from build123d import *

# Parameters (mm, degrees)
Y_KSEKLIK_EKSTR_ZYON1_DEPTH      = 0.1
Y_KSEKLIK_EKSTR_ZYON1_DEPTH_BACK = 16.34
IZIM1_R                          = 1.3
IZIM2_R                          = 2
Y_KSEKLIK_EKSTR_ZYON2_DEPTH      = 0.4
Y_KSEKLIK_EKSTR_ZYON3_START      = 0.4
IZIM3_R                          = 2
Y_KSEKLIK_EKSTR_ZYON3_DEPTH      = 0.4
IZIM4_R                          = 0.45
KES_EKSTR_ZYON1_DEPTH            = 0.5
PAH1_SIZE                        = 0.4
KES_EKSTR_ZYON2_START            = -0.5
IZIM5_R                          = 0.45
KES_EKSTR_ZYON2_DEPTH            = 0.5
PAH2_SIZE                        = 0.4


with BuildPart() as part:
    # Çizim1 → Yükseklik-Ekstrüzyon1 (new, two sides: drawn at the far end of the back side and taken through both)
    with BuildSketch(Plane.XY.offset(-Y_KSEKLIK_EKSTR_ZYON1_DEPTH_BACK)):
        with Locations((3.3, -31.281939442)):
            Circle(IZIM1_R)
    extrude(amount=Y_KSEKLIK_EKSTR_ZYON1_DEPTH + Y_KSEKLIK_EKSTR_ZYON1_DEPTH_BACK)

    # Çizim2 → Yükseklik-Ekstrüzyon2 (add)
    with BuildSketch(Plane.XY.offset(0.1)):
        with Locations((3.3, -31.281939442)):
            Circle(IZIM2_R)
    extrude(amount=Y_KSEKLIK_EKSTR_ZYON2_DEPTH)

    # Çizim3 → Yükseklik-Ekstrüzyon3 (add)
    with BuildSketch(Plane(origin=(0, 0, -16.34), x_dir=(-1, 0, 0), z_dir=(0, 0, -1)).offset(Y_KSEKLIK_EKSTR_ZYON3_START)):
        with Locations(Location((-3.3, -31.281939442, 0), (0, 0, 180))):
            Circle(IZIM3_R)
    extrude(amount=-Y_KSEKLIK_EKSTR_ZYON3_DEPTH)

    # Çizim4 → Kes-Ekstrüzyon1 (cut)
    with BuildSketch(Plane(origin=(0, 0, -16.74), x_dir=(-1, 0, 0), z_dir=(0, 0, -1))):
        with Locations((-3.3, -31.281939442)):
            Circle(IZIM4_R)
    extrude(amount=-KES_EKSTR_ZYON1_DEPTH, mode=Mode.SUBTRACT)

    # Pah1
    pah1_edges = [part.edges().sort_by_distance(p)[0] for p in [
        (3.75, -31.281939442, -16.24),
    ]]
    chamfer(pah1_edges, length=PAH1_SIZE)

    # Çizim5 → Kes-Ekstrüzyon2 (cut)
    with BuildSketch(Plane.XY.offset(0.5).offset(KES_EKSTR_ZYON2_START)):
        with Locations(Location((3.3, -31.281939442, 0), (0, 0, 180))):
            Circle(IZIM5_R)
    extrude(amount=KES_EKSTR_ZYON2_DEPTH, mode=Mode.SUBTRACT)

    # Pah2
    pah2_edges = [part.edges().sort_by_distance(p)[0] for p in [
        (3.75, -31.281939442, 0),
    ]]
    chamfer(pah2_edges, length=PAH2_SIZE)


solid = part.part
Verification items for the finished model (mm, model axes). A direction names the side the tool comes from. Coordinates: 2 decimals unless noted, no trailing zeros. Write each loop counter-clockwise with the first axis right and the second up, starting at its lowest first coordinate (ties: lowest second). Pieces come first, ordered by that corner, then holes. Notation, with made-up numbers: M -5.5,9.25 L 17.5,9.25 A18 cw 17.5,22.25 Z; hole C -36,-7 d3. An arc over 180 degrees is marked long. Use a Markdown table: item, result.
Q1. Sectioned sample at C-C, the plane z = -5.75. Record the boundary of the cut face in (x, y), plus the area to 3 significant figures.
Reply:
| item | result |
|---|---|
| outline | C 3.3,-31.28 d2.6 |
| area | 5.31 mm² |
Q2. Sectioned sample at A-A, the plane y = -29.75. Record the boundary of the cut face in (x, z).
Reply:
| item | result |
|---|---|
| outline | M 2.01,-16.74 L 4.59,-16.74 L 4.59,-16.34 L 2.01,-16.34 Z; M 2.01,0.1 L 4.59,0.1 L 4.59,0.5 L 2.01,0.5 Z |
Q3. Sectioned sample at B-B, the plane x = 2.6. Record the boundary of the cut face in (y, z), plus the area to 3 significant figures.
Reply:
| item | result |
|---|---|
| outline | M -33.16,-16.74 L -29.41,-16.74 L -29.41,-16.34 L -30.19,-16.34 L -30.19,0.1 L -29.41,0.1 L -29.41,0.5 L -33.16,0.5 L -33.16,0.1 L -32.38,0.1 L -32.38,-16.34 L -33.16,-16.34 Z |
| area | 39.0 mm² |
Q4. Sectioned sample at D-D, the plane x = 4.4. Record the boundary of the cut face in (y, z).
Reply:
| item | result |
|---|---|
| outline | M -32.95,-16.74 L -29.61,-16.74 L -29.61,-16.34 L -30.59,-16.34 L -30.59,0.1 L -29.61,0.1 L -29.61,0.5 L -32.95,0.5 L -32.95,0.1 L -31.97,0.1 L -31.97,-16.34 L -32.95,-16.34 Z |
Q5. Thickness scan on line 1 (Z direction, x = 3.35, y = -33.1); line 2 (X direction, y = -31.25, z = -4.75); line 3 (X direction, y = -30.65, z = -12.5). Record the ranges inside material, lowest first.
Reply:
| item | result |
|---|---|
| line 1 | z = -16.74 to -16.34, 0.1 to 0.5 |
| line 2 | x = 2 to 4.6 |
| line 3 | x = 2.16 to 4.44 |
Q6. Set-up check for faces 1 (the face through (3, -32, -16.74)), 2 (the face through (5, -31, -16.34)): record each of +Z, -Z, +X, -X, +Y, -Y from which the full face is reachable in a straight line by a thin tool's end or side.
Reply:
| item | result |
|---|---|
| face 1 | -Z, +X, -X, +Y, -Y |
| face 2 | none |
Q7. Draft check along Z on faces 3 (the face through (4, -32, 0.5)), 4 (the face through (5, -31, 0.1)), 5 (the face through (4.38, -29.6, 0.3)). Enter one of: +Z half, -Z half, draft (parallel to the pull), parting line (faces both ways), or undercut.
Reply:
| item | result |
|---|---|
| face 3 | +Z half |
| face 4 | undercut |
| face 5 | draft |
